```python
from build123d import *

# Parameters (mm, degrees)
F0_R     = 50.1
F0_R_2   = 4.5
F1_DEPTH = 3
F2_R     = 4.5
F3_DEPTH = 25


with BuildPart() as f1:
    # F0 (on Front) → F1 (new body)
    with BuildSketch(Plane.XZ):
        Circle(F0_R)
        Circle(F0_R_2, mode=Mode.SUBTRACT)
    extrude(amount=F1_DEPTH)

    # F2 (on face) → F3 (join)
    with BuildSketch(Plane.XZ.offset(3)):
        Polygon((-4.58071, 8.889156), (-9.98859, 0.477567), (-5.40788, -8.411589), (4.58071, -8.889156), (9.98859, -0.477567), (5.40788, 8.411589), align=None)
        Circle(F2_R, mode=Mode.SUBTRACT)
    extrude(amount=F3_DEPTH)


solid = f1.part
```
Verification items for the finished model (mm, model axes). A direction names the side the tool comes from. Coordinates: 2 decimals unless noted, no trailing zeros. Loops run counter-clockwise (first coordinate to the right, second up) from the corner with the lowest first, then second, coordinate; pieces in that order, holes last. Notation, with made-up numbers: (65, 43) -> (78, 43) arc R7 cw to (78, 48) -> close; hole circle Ø11 at (-25, 45). An arc over 180 degrees is marked (long way). Answer in a Markdown table with one row per item. Add a question column.
1. Material ranges on probe 1 along Y at (x, z) = (27, -29); probe 2 along Z at (x, y) = (0, -21); probe 3 along X at (y, z) = (-2.75, 37), recorded low to high. Write a range as [from, to].
2. Draft check along Z on faces 1 (the face through (-0.484, -15.325, -8.647)), 2 (the face through (-0.59, -13.8, 4.46)), 3 (the face through (-7.25, -15.32, 4.74)). Enter one of: +Z half, -Z half, draft (parallel to the pull), parting line (faces both ways), or undercut.
3. Section check A-A, the plane y = -19.25. Enter the section's corners in (x, z).
4. Section check D-D, the plane x = 13. Enter the section's corners in (y, z), then the cut area to 3 significant figures.
5. Section check C-C, the plane z = -32. Enter the section's corners in (x, y).
6. Depth check by flat-ended pin: P1, Ø8, axis at x = 31, z = -24.5, coming from the -Y side; P2, Ø8, axis at x = -17.5, y = -16.5, coming from the -Z side; P3, Ø10, axis at x = 38.5, z = 21, coming from the +Y side; P4, Ø8, axis at y = -8.5, z = -7.5, coming from the +X side. Enter the tip coordinate at first touch or a pass-through.
7. Section check B-B, the plane x = 0. Enter the section's corners in (y, z), then the cut area to 3 significant figures.
8. Access from +Z, -Z, +X, -X, +Y, -Y to the whole of each face (thin tool, end or side, straight path). Record for faces 4 (the face through (0.484, -15.325, 8.647)), 5 (the face through (-1, 0, -10)), 6 (the face through (7.25, -15.32, -4.74)), 7 (the face through (-7.73, -15.325, -3.905)).
Derived:
| question | item | result |
|---|---|---|
| 1 | probe 1 | y = [-3, 0] |
| 1 | probe 2 | z = [-8.67, -4.5], [4.5, 8.67] |
| 1 | probe 3 | x = [-33.78, 33.78] |
| 2 | face 1 | -Z half |
| 2 | face 2 | undercut |
| 2 | face 3 | +Z half |
| 3 | outline | (-9.99, 0.48) -> (-5.41, -8.41) -> (4.58, -8.89) -> (9.99, -0.48) -> (5.41, 8.41) -> (-4.58, 8.89) -> close; hole circle Ø9 at (0, 0) |
| 4 | outline | (-3, -48.38) -> (0, -48.38) -> (0, 48.38) -> (-3, 48.38) -> close |
| 4 | area | 290 mm² |
| 5 | outline | (-38.55, -3) -> (38.55, -3) -> (38.55, 0) -> (-38.55, 0) -> close |
| 6 | P1 | stops at y = -3 |
| 6 | P2 | passes through |
| 6 | P3 | stops at y = 0 |
| 6 | P4 | stops at x = 8.05 |
| 7 | outline | (-28, -8.67) -> (-3, -8.67) -> (-3, -50.1) -> (0, -50.1) -> (0, -4.5) -> (-28, -4.5) -> close; (-28, 4.5) -> (0, 4.5) -> (0, 50.1) -> (-3, 50.1) -> (-3, 8.67) -> (-28, 8.67) -> close |
| 7 | area | 482 mm² |
| 8 | face 4 | +Z, +X, -Y |
| 8 | face 5 | +Z, -Z, +X, -X, +Y |
| 8 | face 6 | -Z, +X, -Y |
| 8 | face 7 | -Z, -X, -Y |
